```python
from build123d import *

# Parameters (mm, degrees)
F1_DEPTH = 25
F2_W     = 101.8614172935
F2_H     = 6.1345109716
F3_DEPTH = 4
F5_DEPTH = 500


with BuildPart() as f1:
    # F0 (on Front) → F1 (new body)
    with BuildSketch(Plane.XZ):
        Polygon((-62.6290813088, 45.7948409021), (-62.6290813088, 0), (-52.927993238, 0), (-52.927993238, 37.2350551188), (48.9334240556, 37.2350551188), (48.9334240556, 0), (58.6345121264, 0), (58.6345121264, 45.7948409021), align=None)
    extrude(amount=-F1_DEPTH)

    # F2 (on face) → F3 (join)
    with BuildSketch(Plane(origin=(0, 25, 0), x_dir=(-1, 0, 0), z_dir=(0, 1, 0))):
        with Locations((1.9972845912, 3.0672554858)):
            Rectangle(F2_W, F2_H)
    extrude(amount=-F3_DEPTH)

    # F4 (on face) → F5 (cut)
    with BuildSketch(Plane(origin=(-62.6290813088, 0, 0), x_dir=(0, -1, 0), z_dir=(-1, 0, 0))):
        Polygon((-25, 0), (0, 45.7948409021), (-25, 45.7948409021), align=None)
    extrude(amount=-F5_DEPTH, mode=Mode.SUBTRACT)


solid = f1.part
```
CAD build for the part. Positions are in the model's coordinates, mm. A direction names the side the tool comes from. Coordinates: 2 decimals unless noted, no trailing zeros. Order: outer loops, then holes, each group sorted by start corner. A loop starts at its lowest first (then second) coordinate and runs counter-clockwise, first axis right, second up. Notation, with made-up numbers: M 85.25,17 L 117.25,17 A30 ccw 117.25,49 Z; hole C 21,-16.75 d6. An arc over 180 degrees is marked long. Answer as CSV lines item,"result".
1) Cut at C-C (y = 16.25). List the corners of the cut face in (x, z).
Verdict:
outline,"M -62.63,0 L -52.93,0 L -52.93,16.03 L -62.63,16.03 Z; M 48.93,0 L 58.63,0 L 58.63,16.03 L 48.93,16.03 Z"
2) Flat gauge pins, fed straight in: P1, Ø5, axis at x = -30, y = 3.5, coming from the +Z side; P2, Ø1.5, axis at y = 18, z = 13, coming from the +X side; P3, Ø6.5, axis at x = -6, z = 3, coming from the -Y side; P4, Ø1, axis at x = 36.5, y = 3, coming from the +Z side. Where does each tip first touch, or does it go through?
Verdict:
P1,"z = 43.96"
P2,"x = 58.63"
P3,"y = 21"
P4,"z = 41.22"
3) Cut at B-B (z = 21). List the corners of the cut face in (x, y), then the cut area to 3 significant figures.
Verdict:
outline,"M -62.63,0 L -52.93,0 L -52.93,13.54 L -62.63,13.54 Z; M 48.93,0 L 58.63,0 L 58.63,13.54 L 48.93,13.54 Z"
area,"263 mm2"
4) 3-axis set-ups, long thin cutter, end or side, ignore diameter. For faces 4 (the flat face through (-52.928, 8, 14)), 5 (the flat face through (-3, 2, 37.235)), 6 (the flat face through (-3, 0, 38)): which of +Z, -Z, +X, -X, +Y, -Y reach the whole face in a straight line?
Verdict:
face 4,"-Z, -Y"
face 5,"-Z, +Y, -Y"
face 6,"+Z, -Z, +X, -X, -Y"
5) Mould opens along X. For faces 1 (the flat face through (-2.846, 4.342, 37.842)), 2 (the flat face through (-62.629, 7, 13)), 3 (the flat face through (-1, 21, 3)) say: released by +X, released by -X, zero draft, split by the parting line, or undercut.
Verdict:
face 1,"zero draft"
face 2,"released by -X"
face 3,"undercut"
6) Drill centre lines: L1, parallel to X at y = 10, z = 9; L2, parallel to Z at x = 25.5, y = 21.5; L3, parallel to Z at x = 53, y = 18.5. Where is each one in solid material? Low to high. Write a range as from..to.
Verdict:
L1,"-62.63..-52.93, 48.93..58.63"
L2,"0..6.13"
L3,"0..11.91"
7) Cut at A-A (x = 7). List the corners of the cut face in (y, z), then the cut area to 3 significant figures.
Verdict:
outline,"M 0,37.24 L 4.67,37.24 L 0,45.79 Z; M 21,0 L 25,0 L 21.65,6.13 L 21,6.13 Z"
area,"34.3 mm2"
